```python
from build123d import *

# Parameters (mm, degrees)
F1_DEPTH    = 10
F2_T1_DEPTH = 14.1146927807
F3_R        = 0.18


# Not quite as in the source:
# - a fillet or chamfer that OpenCascade refuses, or shapes differently, is made with other operations: its cross-section is extruded or revolved along the edge and cut away or added


with BuildPart() as f1:
    # F0 (on Top) → F1 (new body)
    with BuildSketch(Plane.XY):
        Polygon((10, 0.2012402692), (10, 1), (0.4449767875, 1), (-0.4449767875, 1), (-10, 1), (-10, 0.2012402692), (-0.4449767875, 0.2012402692), (-0.4449767875, -0.2012402692), (-10, -0.2012402692), (-10, -1), (-0.4449767875, -1), (0.4449767875, -1), (10, -1), (10, -0.2012402692), (0.4449767875, -0.2012402692), (0.4449767875, 0.2012402692), align=None)
    extrude(amount=F1_DEPTH)

    # F2: chamfer of 0.8 on 4 edges, made by hand

    # F2_s2 → F2_t1 (cut)
    with BuildSketch(Plane.XY.offset(-2.0573463904)):
        Polygon((-10, -1.0012402692), (-9.2, -0.2012402692), (-10, -0.2012402692), align=None)
        Polygon((-9.2, 0.2012402692), (-10, 1.0012402692), (-10, 0.2012402692), align=None)
        Polygon((9.2, -0.2012402692), (10, -1.0012402692), (10, -0.2012402692), align=None)
        Polygon((10, 1.0012402692), (9.2, 0.2012402692), (10, 0.2012402692), align=None)
    extrude(amount=F2_T1_DEPTH, mode=Mode.SUBTRACT)

    # F3
    f3_edges = [f1.edges().sort_by_distance(p)[0] for p in [
        (-0.444977, -0.20124, 5),
        (-0.444977, 0.20124, 5),
        (0.444977, 0.20124, 5),
        (0.444977, -0.20124, 5),
    ]]
    fillet(f3_edges, radius=F3_R)


solid = f1.part
```
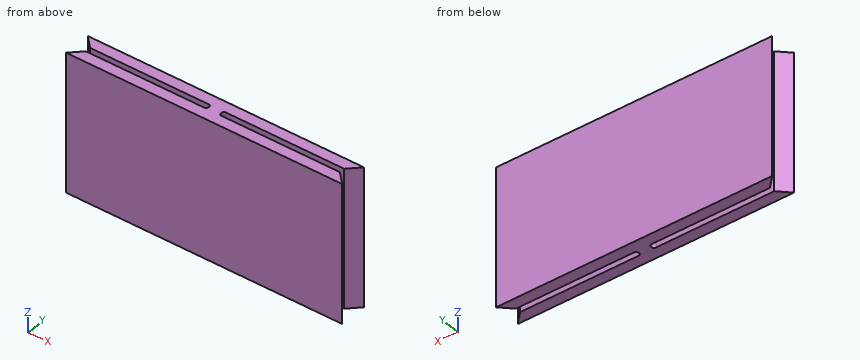
Source: CAD feature listing. Evaluate the final solid. Frame: model axes, mm. Coordinates: 2 decimals unless noted, no trailing zeros. Loops run counter-clockwise (first coordinate to the right, second up) from the corner with the lowest first, then second, coordinate; pieces in that order, holes last. Notation, with made-up numbers: M -24,66.25 L -18,66.25 A33 cw -18,98.25 Z; hole C -20,67 d11. An arc over 180 degrees is marked long. Use CSV: the item, a comma, the result in double quotes.
(1) Cut plane A-A on z = 2. Return loops of the section in (x, y).
Answers follow:
outline,"M -10,-1 L 10,-1 L 9.2,-0.2 L 0.62,-0.2 A0.18 cw 0.44,-0.02 L 0.44,0.02 A0.18 cw 0.62,0.2 L 9.2,0.2 L 10,1 L -10,1 L -9.2,0.2 L -0.62,0.2 A0.18 cw -0.44,0.02 L -0.44,-0.02 A0.18 cw -0.62,-0.2 L -9.2,-0.2 Z"
(2) Line query: line 1 (Y direction, x = 2.75, z = 4.75); line 2 (X direction, y = 0.7, z = 0.75); line 3 (X direction, y = 0.35, z = 9.75). Output: solid intervals per line, ascending. Write a range as [from, to].
Answers follow:
line 1,"[-1, -0.2], [0.2, 1]"
line 2,"[-9.7, 9.7]"
line 3,"[-9.35, 9.35]"
(3) Cut plane B-B on x = -1. Return loops of the section in (y, z).
Answers follow:
outline,"M -1,0 L -0.2,0 L -0.2,10 L -1,10 Z; M 0.2,0 L 1,0 L 1,10 L 0.2,10 Z"
(4) Cut plane C-C on y = 0.4. Return loops of the section in (x, z), and give its area (3 significant figures).
Answers follow:
outline,"M -9.4,0 L 9.4,0 L 9.4,10 L -9.4,10 Z"
area,"188 mm²"
